Can you work these out from the model? Positions are in its coordinate system, mm. A direction names the side the tool comes from. Give positions to 0.01 mm unless a question says otherwise; leave off trailing zeros. Answer as a JSON object with one key per item and string values.
```python
from build123d import *

# Parameters (mm, degrees)
F0_R     = 8.9
F0_R_2   = 2.375
F0_R_3   = 1.95
F1_DEPTH = 5
F2_DEPTH = 2
F3_DEPTH = 2
F4_R     = 5
F5_R     = 1
F6_R     = 2
F7_DEPTH = 12.5
F8_DEPTH = 3


with BuildPart() as f1:
    # F0 (on Right) → F1 (new body)
    with BuildSketch(Plane.YZ):
        with Locations((50, 0)):
            Circle(F0_R)
        with Locations((50, 0)):
            Circle(F0_R_2, mode=Mode.SUBTRACT)
        with Locations((50, 0)):
            Circle(F0_R_2)
        with Locations((50, 0)):
            Circle(F0_R_3, mode=Mode.SUBTRACT)
    extrude(amount=F1_DEPTH)

    # F0 (on Right) → F2 (join)
    with BuildSketch(Plane.YZ):
        with BuildLine():
            ThreePointArc((9.8287842585, -9.8287842585), (12.8419255019, -5.3192997099), (13.9, 0))
            ThreePointArc((13.9, 0), (12.8419255019, 5.3192997099), (9.8287842585, 9.8287842585))
            ThreePointArc((9.8287842585, 9.8287842585), (-13.9, 0), (9.8287842585, -9.8287842585))
        make_face()
        Circle(F0_R, mode=Mode.SUBTRACT)
        with BuildLine():
            ThreePointArc((9.8287842585, 9.8287842585), (12.8419255019, 5.3192997099), (13.9, 0))
            ThreePointArc((13.9, 0), (12.8419255019, -5.3192997099), (9.8287842585, -9.8287842585))
            add(Edge.make_bspline(
                [(9.8287842585, -9.8287842585), (16.2461867133, -7.50000003), (32.6766982829, -7.5000000581), (40.1712157415, -9.8287842585)],
                knots=[0, 0, 0, 0, 30.342431483, 30.342431483, 30.342431483, 30.342431483], degree=3))
            ThreePointArc((40.1712157415, -9.8287842585), (36.1, 0), (40.1712157415, 9.8287842585))
            add(Edge.make_bspline(
                [(9.8287842585, 9.8287842585), (16.2461867454, 7.49999997), (32.6766983239, 7.4999999419), (40.1712157415, 9.8287842585)],
                knots=[0, 0, 0, 0, 30.342431483, 30.342431483, 30.342431483, 30.342431483], degree=3))
        make_face()
        with BuildLine():
            ThreePointArc((63.9, 0), (55.3192997099, 12.8419255019), (40.1712157415, 9.8287842585))
            ThreePointArc((40.1712157415, 9.8287842585), (36.1, 0), (40.1712157415, -9.8287842585))
            ThreePointArc((40.1712157415, -9.8287842585), (55.3192997099, -12.8419255019), (63.9, 0))
        make_face()
        with Locations((50, 0)):
            Circle(F0_R, mode=Mode.SUBTRACT)
    extrude(amount=F2_DEPTH)

    # F0 (on Right) → F3 (join)
    with BuildSketch(Plane.YZ):
        Circle(F0_R)
        Circle(F0_R_2, mode=Mode.SUBTRACT)
        Circle(F0_R_2)
        Circle(F0_R_3, mode=Mode.SUBTRACT)
    extrude(amount=F3_DEPTH)

    # F4
    f4_edges = [f1.edges().sort_by_distance(p)[0] for p in [
        (1, 9.828784, 9.828784),
        (1, 40.171216, 9.828784),
        (1, 9.828784, -9.828784),
        (1, 40.171216, -9.828784),
    ]]
    fillet(f4_edges, radius=F4_R)

    # F5
    f5_edges = [f1.edges().sort_by_distance(p)[0] for p in [
        (2, 63.9, 0),
        (2, 24.980578, 8.083035),
        (2, -13.9, 0),
        (2, 24.980578, -8.083035),
    ]]
    fillet(f5_edges, radius=F5_R)

    # F6 (on Right) → F7 (cut, symmetric)
    with BuildSketch(Plane.YZ):
        with Locations((6, 0)):
            Circle(F6_R)
        with Locations((-6, 0)):
            Circle(F6_R)
        with Locations((0, 6)):
            Circle(F6_R)
        with Locations((0, -6)):
            Circle(F6_R)
    extrude(amount=F7_DEPTH, both=True, mode=Mode.SUBTRACT)

    # F0 (on Right) → F8 (cut)
    with BuildSketch(Plane.YZ):
        with Locations((50, 0)):
            Circle(F0_R_2)
        with Locations((50, 0)):
            Circle(F0_R_3, mode=Mode.SUBTRACT)
    extrude(amount=F8_DEPTH, mode=Mode.SUBTRACT)


solid = f1.part
```
1) Which directions (+Z, -Z, +X, -X, +Y, -Y) give clear straight access to the entire face, cutting with the end or side of a thin tool? Please do faces 1 (the cylindrical face through (3.48, 41.11, 0.39)), 2 (the cylindrical face through (1, 4.4, -1.2)), 3 (the cylindrical face through (1.479, 52.265, 0.713)).
Check sheet entries:
{"face 1": "+X", "face 2": "+X, -X", "face 3": "-X"}
2) I need wall thicknesses on L1, parallel to Z at x = 0.9, y = 0; L2, parallel to Z at x = 4.35, y = 50; L3, parallel to Z at x = 2.6, y = 50 (3 decimals). Which ranges of each line are inside material? Lowest first, please.
Check sheet entries:
{"L1": "-13.9 to -8, -4 to -1.95, 1.95 to 4, 8 to 13.9", "L2": "-8.9 to -1.95, 1.95 to 8.9", "L3": "-8.9 to -2.375, 2.375 to 8.9"}
3) Imagine slicing it at A-A on y = 0. Give the number of separate pieces and of enclosed holes in the cut face, and give its area (3 significant figures).
Check sheet entries:
{"separate pieces": "4", "enclosed holes": "0", "area": "31.4 mm2"}
4) I'm going to push flat-ended pins straight in: P1, Ø4, axis at y = 39.5, z = -6.5, coming from the +X side; P2, Ø3, axis at x = 2, z = 4.5, coming from the -Y side; P3, Ø2, axis at x = 1, z = 10, coming from the -Y side; P4, Ø2.5, axis at y = 0, z = 6, coming from the -X side. Where does each tip first touch, or does it pass through?
Check sheet entries:
{"P1": "x = 2", "P2": "y = -13.5", "P3": "y = -10.59", "P4": "through"}
